The drawing under review shows one solid part. Ordinate dimensions are in mm from its lowest x, y, z. Give positions to 0.01 mm unless a question says otherwise; leave off trailing zeros. Order: outer loops, then holes, each group sorted by start corner. A loop starts at its lowest first (then second) coordinate and runs counter-clockwise, first axis right, second up. Notation, with made-up numbers: (83, 30.5) - (91, 30.5) arc R19 cw to (91, 62.5) - close; hole circle Ø11 at (-7, 18.5). An arc over 180 degrees is marked (long way). Use CSV: the item, a comma, the result in double quotes. Start each with the question number.
1. To check wall thickness, follow line 1 (Y direction, x = 4, z = 2.2); line 2 (X direction, y = 40, z = 2.35) (1 decimal); line 3 (X direction, y = 7, z = 4) (1 decimal). State the ranges of each line that lie inside material, in increasing order. Write a range as [from, to].
2. For pin 1 (1.4 mm diameter, centred on x = 73.5, z = 1.5, fed in from +Y); pin 2 (1.4 mm diameter, centred on y = 34, z = 2, fed in from +X) (1 decimal); pin 3 (1.4 mm diameter, centred on y = 2, z = 3, fed in from -X), all flat-tipped, find the tip position at first contact; note any pin that passes through.
3. Take a section at C-C, the plane y = 28.5. State the section outline as (x, z) points (1 decimal), then the cut area to 3 significant figures.
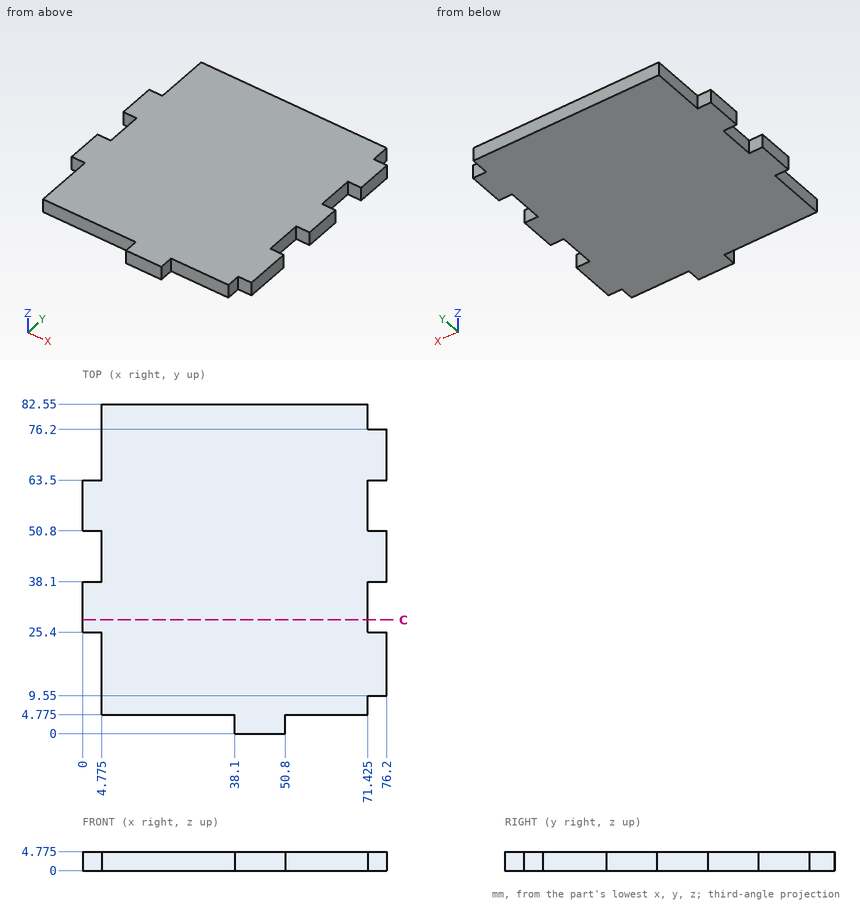
Determined:
1,line 1,"y = [25.4, 38.1], [50.8, 63.5]"
1,line 2,"x = [4.8, 76.2]"
1,line 3,"x = [4.8, 71.4]"
2,pin 1,"stops at y = 76.2"
2,pin 2,"stops at x = 71.4"
2,pin 3,"stops at x = 38.1"
3,outline,"(0, 0) - (71.4, 0) - (71.4, 4.8) - (0, 4.8) - close"
3,area,"341 mm²"
